Geometry: final body of the model. Coordinates: model frame, mm. Coordinates: 2 decimals unless noted, no trailing zeros. Loops run counter-clockwise (first coordinate to the right, second up) from the corner with the lowest first, then second, coordinate; pieces in that order, holes last. Notation, with made-up numbers: (19, -7.75) -> (46, -7.75) arc R15 ccw to (46, -1.75) -> close; hole circle Ø2 at (74, -14.5). An arc over 180 degrees is marked (long way). One line per item, written item: value. Start each with the question number.
Item 1: Section query D-D on z = 3.8. Give the number of separate pieces and of enclosed holes in the cut face, then the cut area to 3 significant figures.
Item 2: Section query B-B on x = 79.5. Return loops of the section in (y, z).
Item 3: Section query C-C on y = -8. Return loops of the section in (x, z), then the cut area to 3 significant figures.
Item 4: Section query A-A on x = -103. Return loops of the section in (y, z).
Item 5: Contact query for flat-ended pins moving along their axis: pin 1 Ø2 at (x, z) = (15, 2.5) entering from -Y; pin 2 Ø2.5 at (y, z) = (68, 3) entering from +X; pin 3 Ø1 at (x, z) = (-100.5, 2.5) entering from +Y. Output: stop coordinate, or through.
Item 6: Ray query, probe 1 along Y at (x, z) = (70.5, 4.65); probe 2 along Y at (x, z) = (110, 2.95); probe 3 along Y at (x, z) = (0, 2.4). Return the intervals inside material, ascending. Write a range as from..to.
Item 7: Mould query, pull axis Y, two halves, no side actions, for faces 1 (the flat face through (2, 84, 5)), 2 (the cylindrical face through (-13.12, -59.06, 2.46)). Classes: +Y half, -Y half, draft (parallel to the pull), parting line (faces both ways), or undercut.
from build123d import *

# Parameters (mm, degrees)
SKETCH1_R           = 60.5
SKETCH1_R_2         = 2.3
BOSS_EXTRUDE1_DEPTH = 5
SKETCH3_W           = 20
SKETCH3_H           = 4.8
CUT_EXTRUDE1_DEPTH  = 5
SKETCH4_W           = 165.999999998
SKETCH4_H           = 5
CUT_EXTRUDE2_DEPTH  = 5
SKETCH5_R           = 2.1
CUT_EXTRUDE3_DEPTH  = 5
SKETCH6_W           = 30
SKETCH6_H           = 5
SKETCH6_W_2         = 150
CUT_EXTRUDE4_DEPTH  = 5
SKETCH7_R           = 2.1
CUT_EXTRUDE5_DEPTH  = 5


with BuildPart() as part:
    # Sketch1 → Boss-Extrude1 (new body)
    with BuildSketch(Plane.XY):
        Polygon((125.000000001, -69.9), (75.000000001, -69.9), (75.000000001, -72.4), (55.000000001, -72.4), (55.000000001, -69.9), (-54.999999999, -69.9), (-54.999999999, -72.4), (-74.999999999, -72.4), (-74.999999999, -69.9), (-124.999999999, -69.9), (-124.999999999, -19.9), (-129.999999999, -19.9), (-129.999999999, 0.1), (-124.999999999, 0.1), (-124.999999999, 110.1), (-129.999999999, 110.1), (-129.999999999, 130.1), (-124.999999999, 130.1), (-124.999999999, 180.1), (125.000000001, 180.1), (125.000000001, 130.1), (130.000000001, 130.1), (130.000000001, 110.1), (125.000000001, 110.1), (125.000000001, 0.1), (130.000000001, 0.1), (130.000000001, -19.9), (125.000000001, -19.9), align=None)
        Circle(SKETCH1_R, mode=Mode.SUBTRACT)
        with Locations((0, -64)):
            Circle(SKETCH1_R_2, mode=Mode.SUBTRACT)
    extrude(amount=BOSS_EXTRUDE1_DEPTH)

    # Sketch3 → Cut-Extrude1 (cut)
    with BuildSketch(Plane.XY.offset(5)):
        with Locations((-102.999999999, 88.505234687)):
            Rectangle(SKETCH3_W, SKETCH3_H)
        with Locations((-102.999999999, 73.505234687)):
            Rectangle(SKETCH3_W, SKETCH3_H)
    cut_extrude1 = extrude(amount=-CUT_EXTRUDE1_DEPTH, mode=Mode.SUBTRACT)

    # Mirror1: Cut-Extrude1 across plane
    add(cut_extrude1.mirror(Plane(origin=(0, 0, 0), x_dir=(0, 0, 1), z_dir=(1, 0, 0))), mode=Mode.SUBTRACT)

    # Sketch4 → Cut-Extrude2 (cut)
    with BuildSketch(Plane.XY.offset(5)):
        with Locations((0, 88.505234687)):
            Rectangle(SKETCH4_W, SKETCH4_H)
        with Locations((0, 73.505234687)):
            Rectangle(SKETCH4_W, SKETCH4_H)
    extrude(amount=-CUT_EXTRUDE2_DEPTH, mode=Mode.SUBTRACT)

    # Sketch5 → Cut-Extrude3 (cut)
    with BuildSketch(Plane.XY.offset(5)):
        with Locations((-109.999999999, -54.9)):
            Circle(SKETCH5_R)
        with Locations((110.000000001, -54.9)):
            Circle(SKETCH5_R)
    extrude(amount=-CUT_EXTRUDE3_DEPTH, mode=Mode.SUBTRACT)

    # Sketch6 → Cut-Extrude4 (cut)
    with BuildSketch(Plane.XY.offset(5)):
        with Locations((-109.999999999, 177.6)):
            Rectangle(SKETCH6_W, SKETCH6_H)
        with Locations((1e-09, 177.6)):
            Rectangle(SKETCH6_W_2, SKETCH6_H)
        with Locations((110.000000001, 177.6)):
            Rectangle(SKETCH6_W, SKETCH6_H)
    extrude(amount=-CUT_EXTRUDE4_DEPTH, mode=Mode.SUBTRACT)

    # Sketch7 → Cut-Extrude5 (cut)
    with BuildSketch(Plane.XY.offset(5)):
        with Locations((-109.999999999, 160.1)):
            Circle(SKETCH7_R)
        with Locations((110.000000001, 160.1)):
            Circle(SKETCH7_R)
    extrude(amount=-CUT_EXTRUDE5_DEPTH, mode=Mode.SUBTRACT)


solid = part.part
Reply:
1. separate pieces: 1
1. enclosed holes: 12
1. area: 48,300 mm²
2. outline: (-69.9, 0) -> (71.01, 0) -> (71.01, 5) -> (-69.9, 5) -> close; (76.01, 0) -> (86.01, 0) -> (86.01, 5) -> (76.01, 5) -> close; (91.01, 0) -> (180.1, 0) -> (180.1, 5) -> (91.01, 5) -> close
3. outline: (-130, 0) -> (-59.97, 0) -> (-59.97, 5) -> (-130, 5) -> close; (59.97, 0) -> (130, 0) -> (130, 5) -> (59.97, 5) -> close
3. area: 700 mm²
4. outline: (-69.9, 0) -> (71.11, 0) -> (71.11, 5) -> (-69.9, 5) -> close; (75.91, 0) -> (86.11, 0) -> (86.11, 5) -> (75.91, 5) -> close; (90.91, 0) -> (175.1, 0) -> (175.1, 5) -> (90.91, 5) -> close
5. pin 1: stops at y = -69.9
5. pin 2: stops at x = 125
5. pin 3: stops at y = 175.1
6. probe 1: y = -72.4..71.01, 76.01..86.01, 91.01..175.1
6. probe 2: y = -69.9..-57, -52.8..71.11, 75.91..86.11, 90.91..158, 162.2..175.1
6. probe 3: y = -69.9..-66.3, -61.7..-60.5, 60.5..71.01, 76.01..86.01, 91.01..175.1
7. face 1: draft
7. face 2: undercut
